For this review, take the finished solid that the model builds, in its own axes (mm). Face numbers are marked on the shaded views. A direction names the side the tool comes from. Round coordinates to 2 decimals unless told otherwise and drop trailing zeros. Loops run counter-clockwise (first coordinate to the right, second up) from the corner with the lowest first, then second, coordinate; pieces in that order, holes last.
1. To check wall thickness, follow line 1 along Z through (x, y) = (13.2, 8); line 2 along Y through (x, z) = (13, 27); line 3 along Z through (x, y) = (13.5, 9.25). State the ranges of each line that lie inside material, in increasing order.
2. Consider section B-B on y = 8. State the section outline as (x, z) points, then the cut area to 3 significant figures.
3. Consider section C-C on z = 13.5. State the section outline as (x, y) points, then the cut area to 3 significant figures.
4. Tool access review of the marked faces 1, 2 and 3: name each direction out of +Z, -Z, +X, -X, +Y, -Y from which nothing blocks a thin tool from reaching the whole face with its end or side.
5. Clearance check with flat-ended pins moving along their axes: pin 1 Ø13 at (x, y) = (-3, 1.5) entering from +Z; pin 2 Ø3.5 at (y, z) = (-8, -22.5) entering from +X; pin 3 Ø3.5 at (y, z) = (8, -22.5) entering from -X. State where each tip first meets the part, or that it passes through.
6. Consider section A-A on z = -22.5. State the section outline as (x, y) points, then the cut area to 3 significant figures.
7. Consider section D-D on y = 0. State the section outline as (x, z) points.
from build123d import *

# Parameters (mm, degrees)
F0_W     = 26
F0_H     = 50
F1_DEPTH = 16
F2_R     = 4
F3_DEPTH = 3
F4_W     = 28
F4_H     = 5
F5_DEPTH = 1320.8
F6_W     = 26
F6_H     = 5
F6_R     = 1.5
F7_DEPTH = 4
F8_R     = 1.5
F9_DEPTH = 4


with BuildPart() as f1:
    # F0 (on Right) → F1 (new body, symmetric)
    with BuildSketch(Plane.YZ):
        Rectangle(F0_W, F0_H)
    extrude(amount=F1_DEPTH, both=True)

    # F2 (on face) → F3 (join)
    with BuildSketch(Plane.YZ.offset(16)):
        with Locations((0, 13.5)):
            Circle(F2_R)
    extrude(amount=F3_DEPTH)

    # F4 (on face) → F5 (cut)
    with BuildSketch(Plane.XZ.offset(13)):
        with Locations((-2, -22.5)):
            Rectangle(F4_W, F4_H)
    extrude(amount=-F5_DEPTH, mode=Mode.SUBTRACT)

    # F6 (on face) → F7 (join)
    with BuildSketch(Plane.YZ.offset(16)):
        with Locations((0, 27.5)):
            Rectangle(F6_W, F6_H)
        with Locations((-8, 27.5)):
            Circle(F6_R, mode=Mode.SUBTRACT)
        with Locations((8, 27.5)):
            Circle(F6_R, mode=Mode.SUBTRACT)
    extrude(amount=-F7_DEPTH)

    # F8 (on face) → F9 (cut)
    with BuildSketch(Plane.YZ.offset(16)):
        with Locations((-8, -22.5)):
            Circle(F8_R)
        with Locations((8, -22.5)):
            Circle(F8_R)
    extrude(amount=-F9_DEPTH, mode=Mode.SUBTRACT)


solid = f1.part
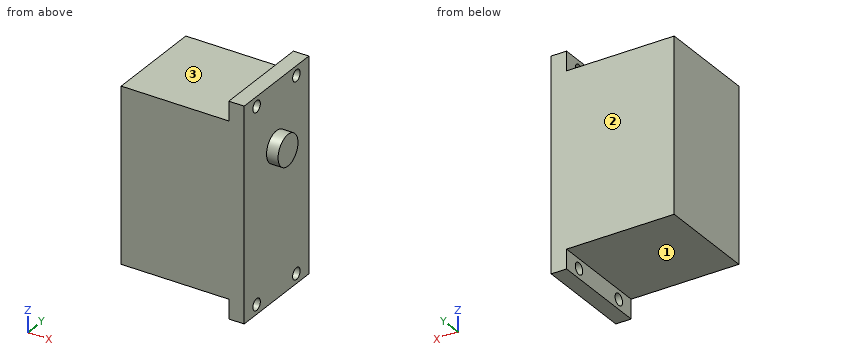
Resolved:
1. line 1: z = -25 to -24, -21 to 26, 29 to 30
1. line 2: y = -13 to -9.41, -6.59 to 6.59, 9.41 to 13
1. line 3: z = -25 to -23.33, -21.67 to 26.67, 28.33 to 30
2. outline: (-16, -20) - (12, -20) - (12, -21) - (16, -21) - (16, 26) - (12, 26) - (12, 25) - (-16, 25) - close; (12, -25) - (16, -25) - (16, -24) - (12, -24) - close; (12, 29) - (16, 29) - (16, 30) - (12, 30) - close
2. area: 1,460 mm2
3. outline: (-16, -13) - (16, -13) - (16, -4) - (19, -4) - (19, 4) - (16, 4) - (16, 13) - (-16, 13) - close
3. area: 856 mm2
4. face 1: -Z, -X, +Y, -Y
4. face 2: +Z, -Z, +X, -X, +Y
4. face 3: +Z, -X, +Y, -Y
5. pin 1: stops at z = 25
5. pin 2: stops at x = 16
5. pin 3: stops at x = 12
6. outline: (12, -13) - (16, -13) - (16, -9.5) - (12, -9.5) - close; (12, -6.5) - (16, -6.5) - (16, 6.5) - (12, 6.5) - close; (12, 9.5) - (16, 9.5) - (16, 13) - (12, 13) - close
6. area: 80.0 mm2
7. outline: (-16, -20) - (12, -20) - (12, -25) - (16, -25) - (16, 9.5) - (19, 9.5) - (19, 17.5) - (16, 17.5) - (16, 30) - (12, 30) - (12, 25) - (-16, 25) - close
